from build123d import *

# Parameters (mm, degrees)
EXTRUDE_1_DEPTH     = 10
SKETCH_2_R          = 8
CUT_EXTRUDE_1_DEPTH = 20
CHAMFER_1_SIZE      = 1
SKETCH_3_OUTSIDE_W  = 130.214
SKETCH_3_OUTSIDE_H  = 126.192
SKETCH_3_OUTSIDE_R  = 13
CUT_EXTRUDE_2_DEPTH = 45
CUT_EXTRUDE_2_DRAFT = -45
SKETCH_4_OUTSIDE_W  = 130.214
SKETCH_4_OUTSIDE_H  = 126.192
SKETCH_4_OUTSIDE_R  = 13
CUT_EXTRUDE_3_DEPTH = 45
CUT_EXTRUDE_3_DRAFT = -45


with BuildPart() as part:
    # 草图1 → 凸台-拉伸1 (new body)
    with BuildSketch(Plane(origin=(0, 0, 0), x_dir=(0, 0, -1), z_dir=(1, 0, 0))):
        Polygon((-7.505553499, -13), (7.505553499, -13), (15.011106999, 0), (7.505553499, 13), (-7.505553499, 13), (-15.011106999, 0), align=None)
    extrude(amount=EXTRUDE_1_DEPTH)

    # 草图2 → 切除-拉伸1 (cut)
    with BuildSketch(Plane(origin=(10, 0, 0), x_dir=(0, 0, -1), z_dir=(1, 0, 0))):
        Circle(SKETCH_2_R)
    extrude(amount=-CUT_EXTRUDE_1_DEPTH, mode=Mode.SUBTRACT)

    # 倒角1
    chamfer_1_edges = [part.edges().sort_by_distance(p)[0] for p in [
        (0, 0, 8),
        (10, 0, 8),
    ]]
    chamfer(chamfer_1_edges, length=CHAMFER_1_SIZE)


with BuildPart() as cut_extrude_2_tool:
    # 草图3 outside → 切除-拉伸2 (with draft: the straight prism first)
    with BuildSketch(Plane(origin=(10, 0, 0), x_dir=(0, 0, -1), z_dir=(1, 0, 0))):
        Rectangle(SKETCH_3_OUTSIDE_W, SKETCH_3_OUTSIDE_H)
        Circle(SKETCH_3_OUTSIDE_R, mode=Mode.SUBTRACT)
    extrude(amount=-CUT_EXTRUDE_2_DEPTH)
    # 切除-拉伸2: the draft: its side faces are tilted about the plane it starts from
    cut_extrude_2_sides = [cut_extrude_2_tool.faces().sort_by_distance(p)[0] for p in [
        (-12.5, -63.096, 0),
        (-12.5, 0, -65.107),
        (-12.5, 63.096, 0),
        (-12.5, 0, 65.107),
        (-12.5, 0, 13),
    ]]
    draft(cut_extrude_2_sides, Plane(origin=(10, 0, 0), x_dir=(0, 0, -1), z_dir=(1, 0, 0)), CUT_EXTRUDE_2_DRAFT)


with BuildPart() as part_1:
    add(part.part)

    # 切除-拉伸2: cut by cut_extrude_2_tool
    add(cut_extrude_2_tool.part, mode=Mode.SUBTRACT)


with BuildPart() as cut_extrude_3_tool:
    # 草图4 outside → 切除-拉伸3 (with draft: the straight prism first)
    with BuildSketch(Plane.ZY):
        Rectangle(SKETCH_4_OUTSIDE_W, SKETCH_4_OUTSIDE_H)
        Circle(SKETCH_4_OUTSIDE_R, mode=Mode.SUBTRACT)
    extrude(amount=-CUT_EXTRUDE_3_DEPTH)
    # 切除-拉伸3: the draft: its side faces are tilted about the plane it starts from
    cut_extrude_3_sides = [cut_extrude_3_tool.faces().sort_by_distance(p)[0] for p in [
        (22.5, -63.096, 0),
        (22.5, 0, 65.107),
        (22.5, 63.096, 0),
        (22.5, 0, -65.107),
        (22.5, 0, -13),
    ]]
    draft(cut_extrude_3_sides, Plane.ZY, CUT_EXTRUDE_3_DRAFT)


with BuildPart() as part_2:
    add(part_1.part)

    # 切除-拉伸3: cut by cut_extrude_3_tool
    add(cut_extrude_3_tool.part, mode=Mode.SUBTRACT)


solid = part_2.part
Can you work these out from the model? Positions are in its coordinate system, mm. Give positions to 0.01 mm unless a question says otherwise; leave off trailing zeros. Loops run counter-clockwise (first coordinate to the right, second up) from the corner with the lowest first, then second, coordinate; pieces in that order, holes last. Notation, with made-up numbers: (-11, 60) -> (46, 60) arc R21 cw to (46, 95) -> close; hole circle Ø1 at (45, 52). An arc over 180 degrees is marked (long way). Use one line per item in the form item = value.
1) We'd pull the mould along Y, two halves only. Please class faces 1 (the face through (5.06, -7.81, 1.73)), 2 (the face through (9.521, -11.657, 6.768)), 3 (the face through (5, 13, 0)): released by +Y, released by -Y, zero draft, split by the parting line, or undercut.
Answers:
face_1 = undercut
face_2 = released by -Y
face_3 = released by +Y
2) Will these pins go through, and if not, where does the flat tip stop? pin 1 (1.5 mm diameter, centred on x = 5, y = 5.5, fed in from +Z); pin 2 (2 mm diameter, centred on x = 5, y = 2.5, fed in from -Z); pin 3 (6 mm diameter, centred on x = 7, y = 7.5, fed in from -Z).
Answers:
pin_1 = 12.27
pin_2 = -14.15
pin_3 = -12.41
3) If we section it at A-A (x = 4): Please give me the cut outline in (y, z).
Answers:
outline = (-13, -7.51) -> (0, -15.01) -> (13, -7.51) -> (13, 7.51) -> (0, 15.01) -> (-13, 7.51) -> close; hole circle Ø16 at (0, 0)
4) I need wall thicknesses on line 1 along Y through (x, z) = (7.25, 0); line 2 along Z through (x, y) = (8.75, 5.75); line 3 along Y through (x, z) = (4, 2.5). Which ranges of each line are inside material? Lowest first, please.
Answers:
line_1 = -13 to -8, 8 to 13
line_2 = -11.69 to -5.56, 5.56 to 11.69
line_3 = -13 to -7.6, 7.6 to 13
